Design review of the part shown in the three views and the two pictorial views. Dimensions are in mm from the part's minimum x, y and z. Round coordinates to 2 decimals unless told otherwise and drop trailing zeros. Order: outer loops, then holes, each group sorted by start corner. A loop starts at its lowest first (then second) coordinate and runs counter-clockwise, first axis right, second up. Notation, with made-up numbers: (-33.75, 32.25) -> (3.25, 32.25) arc R15 ccw to (3.25, 54.25) -> close; hole circle Ø6 at (36.5, -38.75). An arc over 180 degrees is marked (long way). Put each result on its own line as item: value. Start each with the question number.
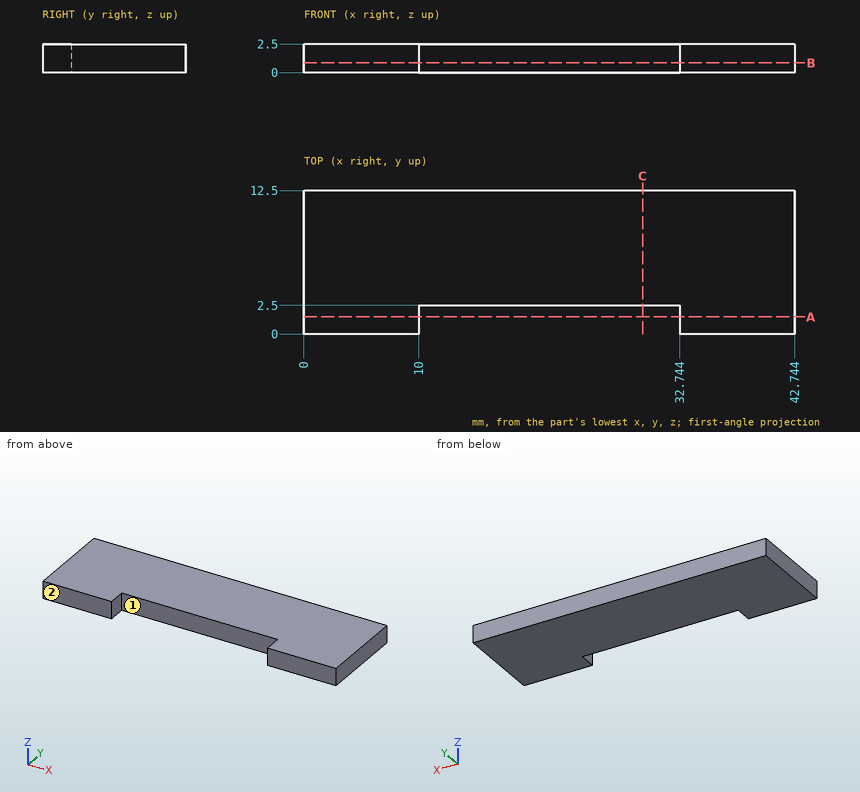
Q1. Take a section at B-B on z = 0.85. Give the boundary of the cut face in (x, y).
Q2. Take a section at A-A on y = 1.5. Give the boundary of the cut face in (x, z).
Q3. Wall thickness on probe 1 along X at (y, z) = (1.25, 0.9); probe 2 along Y at (x, z) = (18, 1.3): over which ranges is each line inside the solid? List them lowest first. Write a range as [from, to].
Q4. Take a section at C-C on x = 29.5. Give the boundary of the cut face in (y, z).
Q5. Draft analysis for pull direction X (two halves, no side actions). For the marked faces 1 and 2, state which applies: +X half, -X half, draft (parallel to the pull), parting line (faces both ways), or undercut.
Calculated:
1. outline: (0, 0) -> (10, 0) -> (10, 2.5) -> (32.74, 2.5) -> (32.74, 0) -> (42.74, 0) -> (42.74, 12.5) -> (0, 12.5) -> close
2. outline: (0, 0) -> (10, 0) -> (10, 2.5) -> (0, 2.5) -> close; (32.74, 0) -> (42.74, 0) -> (42.74, 2.5) -> (32.74, 2.5) -> close
3. probe 1: x = [0, 10], [32.74, 42.74]
3. probe 2: y = [2.5, 12.5]
4. outline: (2.5, 0) -> (12.5, 0) -> (12.5, 2.5) -> (2.5, 2.5) -> close
5. face 1: undercut
5. face 2: draft
